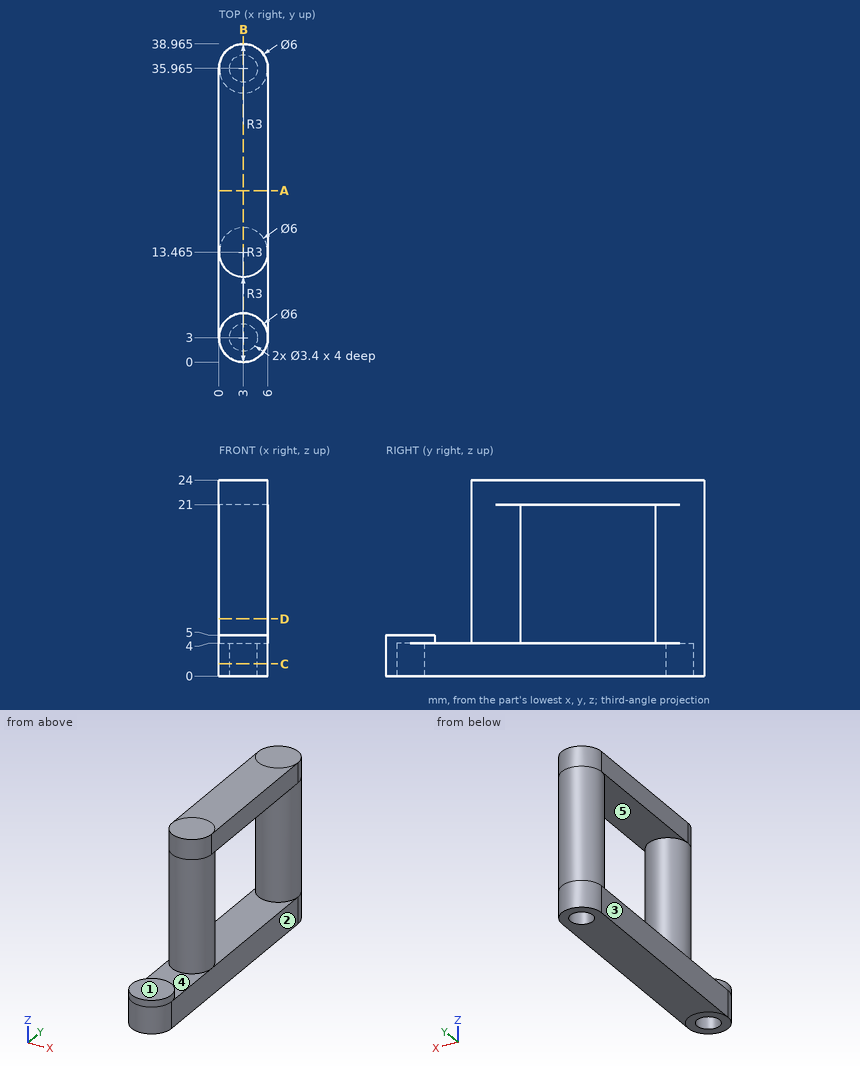
Check sheet for the drawn part. Datum: minimum x, y, z corner. Units: mm. A direction names the side the tool comes from. Round coordinates to 2 decimals unless told otherwise and drop trailing zeros. Loops run counter-clockwise (first coordinate to the right, second up) from the corner with the lowest first, then second, coordinate; pieces in that order, holes last.
Item 1: Cross-section at D-D on z = 7. Record the boundary of the cut face in (x, y) (1 decimal).
Item 2: Cross-section at A-A on y = 21. Record the boundary of the cut face in (x, z), then the cut area to 3 significant figures.
Item 3: Gauge pin test, flat ends, axial feed: pin 1 (1 mm diameter, centred on x = 5, z = 20, fed in from -Y); pin 2 (3 mm diameter, centred on x = 3, y = 3, fed in from -Z); pin 3 (6 mm diameter, centred on y = 16, z = 10, fed in from +X); pin 4 (1 mm diameter, centred on x = 2.5, z = 11.5, fed in from -Y) (3 decimals). Record the tip position at first contact, or that the pin passes through.
Item 4: Mould release check, pull along Z, two halves, no side actions. Record for the marked faces 3, 4 and 5: pulls with the +Z half, pulls with the -Z half, needs draft (parallel to the pull), parting line crosses it, or undercut.
Item 5: Access from +Z, -Z, +X, -X, +Y, -Y to the whole of each face (thin tool, end or side, straight path). Record for the marked faces 1 and 2.
Item 6: Cross-section at B-B on x = 3. Record the boundary of the cut face in (y, z) (1 decimal), then the cut area to 3 significant figures.
Item 7: Cross-section at C-C on z = 1.5. Record the boundary of the cut face in (x, y) (1 decimal), then the cut area to 3 significant figures.
Item 8: Thickness scan on line 1 (Y direction, x = 3, z = 1.6) (1 decimal); line 2 (Z direction, x = 2.95, y = 30); line 3 (X direction, y = 3, z = 1.4). Record the ranges inside material, lowest first.
Answer sheet:
1. outline: circle Ø6 at (3, 13.5); circle Ø6 at (3, 36)
2. outline: (0, 0) - (6, 0) - (6, 4) - (0, 4) - close; (0, 21) - (6, 21) - (6, 24) - (0, 24) - close
2. area: 42.0 mm2
3. pin 1: stops at y = 10.87
3. pin 2: stops at z = 4
3. pin 3: stops at x = 6
3. pin 4: stops at y = 10.465
4. face 3: needs draft
4. face 4: pulls with the +Z half
4. face 5: undercut
5. face 1: +Z, +X, -X, -Y
5. face 2: +Z, -Z, +X, +Y, -Y
6. outline: (0, 0) - (1.3, 0) - (1.3, 4) - (4.7, 4) - (4.7, 0) - (34.3, 0) - (34.3, 4) - (37.7, 4) - (37.7, 0) - (39, 0) - (39, 24) - (10.5, 24) - (10.5, 4) - (6, 4) - (6, 5) - (0, 5) - close; hole (16.5, 4) - (33, 4) - (33, 21) - (16.5, 21) - close
6. area: 424 mm2
7. outline: (0, 3) arc R3 ccw to (6, 3) - (6, 36) arc R3 ccw to (0, 36) - close; hole circle Ø3.4 at (3, 3); hole circle Ø3.4 at (3, 36)
7. area: 208 mm2
8. line 1: y = 0 to 1.3, 4.7 to 34.3, 37.7 to 39
8. line 2: z = 0 to 4, 21 to 24
8. line 3: x = 0 to 1.3, 4.7 to 6
